For this review, take the finished solid that the model builds, in its own axes (mm). A direction names the side the tool comes from. Coordinates: 2 decimals unless noted, no trailing zeros. Write each loop counter-clockwise with the first axis right and the second up, starting at its lowest first coordinate (ties: lowest second). Pieces come first, ordered by that corner, then holes. Notation, with made-up numbers: (12, 50) - (29, 50) arc R28 cw to (29, 89) - close; hole circle Ø9 at (-8, 54.5). An arc over 180 degrees is marked (long way). Use one line per item in the form item = value. Start each with the question number.
1) We need section B-B (x = -47). Give the boundary of the cut face in (y, z) (3 decimals), plus the area to 3 significant figures.
2) For L1, parallel to X at y = 147, z = 1.5; L2, parallel to X at y = 124.5, z = 2.3; L3, parallel to X at y = 75, z = 2.4, list the stretches that pass through material, from the lowest coordinate up. Write a range as from..to.
3) We need section C-C (z = 2.2). Count the separate pieces of the cut face and the enclosed holes in it, plus the area to 3 significant figures.
4) Insertion check: P1, Ø1.9, axis at x = 77.79, y = 64.54, coming from the -Z side; P2, Ø1, axis at x = 28.5, z = 1.5, coming from the +Y side; P3, Ø1.5, axis at x = 28.5, z = 1, coming from the +Y side; P4, Ø1.6, axis at y = 113, z = 1, coming from the -X side. Each pin has a flat end and moves straight along its axis. Give the tip position at first contact, or say it passes through.
5) Mouldability with a two-part tool opening along Y and no side actions: class faces 1 (the cylindrical face through (-0.413, 175.634, 1.565)), 2 (the cylindrical face through (0.385, 197.883, 1.565)), 3 (the cylindrical face through (-27.408, 56.375, 1.565)), 4 (the flat face through (-1, 102, 3.175)) as pulls with the +Y half, pulls with the -Y half, needs draft (parallel to the pull), parting line crosses it, or undercut.
6) We need section A-A (y = 118.5). Give the boundary of the cut face in (x, z) (3 decimals).
7) Tool access review of faces 5 (the cylindrical face through (27.112, 56.276, 1.565)), 6 (the cylindrical face through (14.511, 82.955, 1.565)): name each direction out of +Z, -Z, +X, -X, +Y, -Y from which nothing blocks a thin tool from reaching the whole face with its end or side.
8) We need section D-D (y = 154). Give the boundary of the cut face in (x, z) (3 decimals), plus the area to 3 significant figures.
```python
from build123d import *

# Parameters (mm, degrees)
SKETCH5_R           = 1.5875
SKETCH5_R_2         = 3.175
BOSS_EXTRUDE2_DEPTH = 3.175


with BuildPart() as part:
    # Sketch5 → Boss-Extrude2 (new body)
    with BuildSketch(Plane.XY):
        with BuildLine():
            Line((-82.55, 70.885609673), (-82.55, 58.185609673))
            Line((-82.55, 58.185609673), (-31.848963051, 58.185609673))
            ThreePointArc((-31.848963051, 58.185609673), (-27.35883499, 56.325737733), (-25.498963051, 51.835609673))
            Line((-25.498963051, 51.835609673), (-25.498963051, 42.310609673))
            ThreePointArc((-25.498963051, 42.310609673), (-24.569027081, 40.065545642), (-22.323963051, 39.135609673))
            Line((-22.323963051, 39.135609673), (22.126036949, 39.135609673))
            ThreePointArc((22.126036949, 39.135609673), (24.37110098, 40.065545642), (25.301036949, 42.310609673))
            Line((25.301036949, 42.310609673), (25.301036949, 51.835609673))
            ThreePointArc((25.301036949, 51.835609673), (27.160908889, 56.325737733), (31.651036949, 58.185609673))
            Line((31.651036949, 58.185609673), (82.55, 58.185609673))
            Line((82.55, 58.185609673), (82.55, 70.885609673))
            Line((82.55, 70.885609673), (22.446426721, 184.373331383))
            ThreePointArc((22.446426721, 184.373331383), (0, 197.885609673), (-22.446426721, 184.373331383))
            Line((-22.446426721, 184.373331383), (-82.55, 70.885609673))
        make_face()
        with Locations((-77.7875, 64.535609673)):
            Circle(SKETCH5_R, mode=Mode.SUBTRACT)
        with Locations((77.7875, 64.535609673)):
            Circle(SKETCH5_R, mode=Mode.SUBTRACT)
        with Locations((-21.166666667, 47.762966307)):
            Circle(SKETCH5_R, mode=Mode.SUBTRACT)
        with Locations((21.166666667, 47.762966307)):
            Circle(SKETCH5_R, mode=Mode.SUBTRACT)
        with Locations((0, 172.485609673)):
            Circle(SKETCH5_R_2, mode=Mode.SUBTRACT)
        with BuildLine():
            Line((-57.861180964, 90.3675401), (-28.80539088, 145.230757697))
            ThreePointArc((-28.80539088, 145.230757697), (-24.546211379, 148.463135508), (-19.3281535, 147.296624336))
            ThreePointArc((-19.3281535, 147.296624336), (-17.639343437, 146.086441824), (-15.875, 144.989303103))
            ThreePointArc((-15.875, 144.989303103), (-13.550738686, 142.665041789), (-12.7, 139.490041789))
            Line((-12.7, 139.490041789), (-12.7, 87.395609673))
            ThreePointArc((-12.7, 87.395609673), (-14.559871939, 82.905481612), (-19.05, 81.045609673))
            Line((-19.05, 81.045609673), (-52.249574284, 81.045609673))
            ThreePointArc((-52.249574284, 81.045609673), (-57.689898641, 84.120648468), (-57.861180964, 90.3675401))
        make_face(mode=Mode.SUBTRACT)
        with BuildLine():
            Line((57.861180964, 90.3675401), (28.80539088, 145.230757697))
            ThreePointArc((28.80539088, 145.230757697), (24.546211379, 148.463135508), (19.3281535, 147.296624336))
            ThreePointArc((19.3281535, 147.296624336), (17.639343437, 146.086441824), (15.875, 144.989303103))
            ThreePointArc((15.875, 144.989303103), (13.550738686, 142.665041789), (12.7, 139.490041789))
            Line((12.7, 139.490041789), (12.7, 87.395609673))
            ThreePointArc((12.7, 87.395609673), (14.559871939, 82.905481612), (19.05, 81.045609673))
            Line((19.05, 81.045609673), (52.249574284, 81.045609673))
            ThreePointArc((52.249574284, 81.045609673), (57.689898641, 84.120648468), (57.861180964, 90.3675401))
        make_face(mode=Mode.SUBTRACT)
        with BuildLine():
            Line((-11.2, 64.474125728), (-11.2, 77.174125728))
            ThreePointArc((-11.2, 77.174125728), (-9.5, 78.874125728), (-7.8, 77.174125728))
            Line((-7.8, 77.174125728), (-7.8, 64.474125728))
            ThreePointArc((-7.8, 64.474125728), (-9.5, 62.774125728), (-11.2, 64.474125728))
        make_face(mode=Mode.SUBTRACT)
        with BuildLine():
            Line((-1.7, 56.474125728), (-1.7, 85.174125728))
            ThreePointArc((-1.7, 85.174125728), (0, 86.874125728), (1.7, 85.174125728))
            Line((1.7, 85.174125728), (1.7, 56.474125728))
            ThreePointArc((1.7, 56.474125728), (0, 54.774125728), (-1.7, 56.474125728))
        make_face(mode=Mode.SUBTRACT)
        with BuildLine():
            Line((7.8, 64.474125728), (7.8, 77.174125728))
            ThreePointArc((7.8, 77.174125728), (9.5, 78.874125728), (11.2, 77.174125728))
            Line((11.2, 77.174125728), (11.2, 64.474125728))
            ThreePointArc((11.2, 64.474125728), (9.5, 62.774125728), (7.8, 64.474125728))
        make_face(mode=Mode.SUBTRACT)
    extrude(amount=BOSS_EXTRUDE2_DEPTH)


solid = part.part
```
Determined:
q1.outline = (58.186, 0) - (81.046, 0) - (81.046, 3.175) - (58.186, 3.175) - close; (110.876, 0) - (138.011, 0) - (138.011, 3.175) - (110.876, 3.175) - close
q1.area = 159 mm²
q2.L1 = -42.24..-27.42, -18.94..18.94, 27.42..42.24
q2.L2 = -54.16..-39.78, -12.7..12.7, 39.78..54.16
q2.L3 = -80.37..-11.2, -7.8..-1.7, 1.7..7.8, 11.2..80.37
q3.separate_pieces = 1
q3.enclosed_holes = 10
q3.area = 10,900 mm²
q4.P1 = through
q4.P2 = 173.89
q4.P3 = 174.36
q4.P4 = -60.67
q5.face_1 = undercut
q5.face_2 = pulls with the +Y half
q5.face_3 = pulls with the -Y half
q5.face_4 = needs draft
q6.outline = (-57.333, 0) - (-42.962, 0) - (-42.962, 3.175) - (-57.333, 3.175) - close; (-12.7, 0) - (12.7, 0) - (12.7, 3.175) - (-12.7, 3.175) - close; (42.962, 0) - (57.333, 0) - (57.333, 3.175) - (42.962, 3.175) - close
q7.face_5 = +Z, -Z, +X, -Y
q7.face_6 = +Z, -Z
q8.outline = (-38.532, 0) - (38.532, 0) - (38.532, 3.175) - (-38.532, 3.175) - close
q8.area = 245 mm²
